Geometry: final body of the model. Coordinates: model frame, mm. Coordinates: 2 decimals unless noted, no trailing zeros. Loops run counter-clockwise (first coordinate to the right, second up) from the corner with the lowest first, then second, coordinate; pieces in that order, holes last. Notation, with made-up numbers: (80, 31.25) - (127, 31.25) arc R26 ccw to (127, 49.25) - close; hole circle Ø3 at (51, -27.5). An arc over 180 degrees is marked (long way). Answer in a Markdown table with one row per item.
from build123d import *

# Parameters (mm, degrees)
SKETCH_8_R               = 5.2
EXTRUDE_4_DEPTH          = 2.5
CUT_EXTRUDE_8_DEPTH      = 2.5
CUT_EXTRUDE_8_DEPTH_BACK = 2.5
SKETCH_11_R              = 5
CUT_EXTRUDE_9_DEPTH      = 2.5
CUT_EXTRUDE_9_DEPTH_BACK = 2.5
SKETCH_12_W              = 11.101506765
SKETCH_12_H              = 17.426783875


with BuildPart() as part:
    # Sketch 8 → Extrude 4 (new body)
    with BuildSketch(Plane(origin=(0, 0, 0), x_dir=(1, 0, 0), z_dir=(0, 1, 0))):
        with Locations(Location((0, 0, 0), (0, 0, 270))):
            Circle(SKETCH_8_R)
    extrude(amount=EXTRUDE_4_DEPTH)

    # Sketch 11 → Cut-Extrude 8 (cut, two sides: drawn at the far end of the back side and taken through both)
    with BuildSketch(Plane(origin=(0, 0, 0), x_dir=(1, 0, 0), z_dir=(0, 1, 0)).offset(-CUT_EXTRUDE_8_DEPTH_BACK)):
        with Locations(Location((0, 0, 0), (0, 0, 270))):
            Circle(SKETCH_11_R)
    extrude(amount=CUT_EXTRUDE_8_DEPTH + CUT_EXTRUDE_8_DEPTH_BACK, mode=Mode.SUBTRACT)

    # Sketch 12 → Cut-Extrude 9 (cut, two sides: drawn at the far end of the back side and taken through both)
    with BuildSketch(Plane(origin=(0, 0, 0), x_dir=(1, 0, 0), z_dir=(0, 1, 0)).offset(-CUT_EXTRUDE_9_DEPTH_BACK)):
        with Locations((5.550753382, -1.742678388)):
            Rectangle(SKETCH_12_W, SKETCH_12_H)
    extrude(amount=CUT_EXTRUDE_9_DEPTH + CUT_EXTRUDE_9_DEPTH_BACK, mode=Mode.SUBTRACT)


solid = part.part
(1) Cut plane A-A on x = -0.6. Output: boundary loops of the cut face in (y, z).
Verdict:
| item | result |
|---|---|
| outline | (0, -5.17) - (2.5, -5.17) - (2.5, -4.96) - (0, -4.96) - close; (0, 4.96) - (2.5, 4.96) - (2.5, 5.17) - (0, 5.17) - close |
(2) First-contact query: pin 1 Ø1.5 at (y, z) = (1.5, 2.5) entering from -X. Flat tip, straight axial feed; report the tip coordinate or a pass-through.
Verdict:
| item | result |
|---|---|
| pin 1 | stops at x = -4.9 |
(3) Cut plane D-D on x = -4.4. Output: boundary loops of the cut face in (y, z).
Verdict:
| item | result |
|---|---|
| outline | (0, -2.77) - (2.5, -2.77) - (2.5, -2.37) - (0, -2.37) - close; (0, 2.37) - (2.5, 2.37) - (2.5, 2.77) - (0, 2.77) - close |
(4) Cut plane B-B on y = 2. Output: boundary loops of the cut face in (x, z), then the cut area to 3 significant figures.
Verdict:
| item | result |
|---|---|
| outline | (0, -5.2) - (0, -5) arc R5 cw to (0, 5) - (0, 5.2) arc R5.2 ccw to start |
| area | 3.20 mm² |
(5) Cut plane C-C on z = 0. Output: boundary loops of the cut face in (x, y), then the cut area to 3 significant figures.
Verdict:
| item | result |
|---|---|
| outline | (-5.2, 0) - (-5, 0) - (-5, 2.5) - (-5.2, 2.5) - close |
| area | 0.500 mm² |
(6) Ray query, probe 1 along Z at (x, y) = (-3.4, 1.75); probe 2 along Z at (x, y) = (-3.35, 1.6); probe 3 along X at (y, z) = (0.3, 2). Return the intervals inside material, ascending.
Verdict:
| item | result |
|---|---|
| probe 1 | z = -3.93 to -3.67, 3.67 to 3.93 |
| probe 2 | z = -3.98 to -3.71, 3.71 to 3.98 |
| probe 3 | x = -4.8 to -4.58 |
(7) Pull-direction query (Z, two-part tool) for faces 1 (the face through (-5, 1, 0)), 2 (the face through (-5.2, 1.2, -0.1)); classes: pulls with the +Z half, pulls with the -Z half, needs draft (parallel to the pull), parting line crosses it, or undercut.
Verdict:
| item | result |
|---|---|
| face 1 | undercut |
| face 2 | parting line crosses it |
